Source: CAD feature listing. Evaluate the final solid. Frame: model axes, mm. A direction names the side the tool comes from. Round coordinates to 2 decimals unless told otherwise and drop trailing zeros. Loops run counter-clockwise (first coordinate to the right, second up) from the corner with the lowest first, then second, coordinate; pieces in that order, holes last. Notation, with made-up numbers: M -27,-9.5 L -22,-9.5 A23 cw -22,-0.5 Z; hole C 31.25,64.25 d6. An arc over 180 degrees is marked long. Answer as a JSON object with one key per item and string values.
from build123d import *

# Parameters (mm, degrees)
SKETCH_1_R      = 3
EXTRUDE_1_DEPTH = 5
SKETCH_2_R      = 3
EXTRUDE_2_DEPTH = 5


with BuildPart() as part:
    # 草图1 → 凸台-拉伸1 (new body)
    with BuildSketch(Plane(origin=(0, 0, 0), x_dir=(1, 0, 0), z_dir=(0, 1, 0))):
        with BuildLine():
            Line((-92.110125605, 6.217636835), (157.889874395, 6.217636835))
            ThreePointArc((157.889874395, 6.217636835), (162.889874395, 1.217636835), (157.889874395, -3.782363165))
            Line((157.889874395, -3.782363165), (-92.110125605, -3.782363165))
            ThreePointArc((-92.110125605, -3.782363165), (-97.110125605, 1.217636835), (-92.110125605, 6.217636835))
        make_face()
        with Locations(Location((-92.110125605, 1.217636835, 0), (0, 0, 270))):
            Circle(SKETCH_1_R, mode=Mode.SUBTRACT)
    extrude(amount=EXTRUDE_1_DEPTH)

    # 草图2 → 凸台-拉伸2 (add)
    with BuildSketch(Plane(origin=(0, 5, 0), x_dir=(1, 0, 0), z_dir=(0, 1, 0))):
        with Locations(Location((157.889874395, 1.217636835, 0), (0, 0, 270))):
            Circle(SKETCH_2_R)
    extrude(amount=EXTRUDE_2_DEPTH)


solid = part.part
Item 1: Contact query for a flat-ended pin moving along its axis: pin 1 Ø1 at (x, z) = (126, -0.5) entering from +Y. Output: stop coordinate, or through.
Answer sheet:
{"pin 1": "stops at y = 5"}
Item 2: Pull-direction query (Z, two-part tool) for faces 3 (the flat face through (158, 10, -1)), 4 (the flat face through (31, 2, -6.218)), 5 (the cylindrical face through (-93.936, 2.465, -3.598)); classes: pulls with the +Z half, pulls with the -Z half, needs draft (parallel to the pull), parting line crosses it, or undercut.
Answer sheet:
{"face 3": "needs draft", "face 4": "pulls with the -Z half", "face 5": "undercut"}
Item 3: Access query for faces 1 (the cylindrical face through (160.419, 7.465, 0.395)), 2 (the flat face through (35, 2, 3.782)). Directions: +Z, -Z, +X, -X, +Y, -Y. A direction counts if a zero-diameter tool reaches every point of the face in a straight line with its end or side. Return the directions, or none.
Answer sheet:
{"face 1": "+Y", "face 2": "+Z, +X, -X, +Y, -Y"}
Item 4: Section A-A on y = 3.25. Return the cut outline in (x, z).
Answer sheet:
{"outline": "M -92.11,-6.22 L 157.89,-6.22 A5 ccw 157.89,3.78 L -92.11,3.78 A5 ccw Z; hole C -92.11,-1.22 d6"}
Item 5: Line query: probe 1 along Y at (x, z) = (-48.5, 2.75); probe 2 along X at (y, z) = (1, -3.75); probe 3 along X at (y, z) = (2.25, -2.75). Output: solid intervals per line, ascending. Write a range as from..to.
Answer sheet:
{"probe 1": "y = 0..5", "probe 2": "x = -96.42..-93.72, -90.5..162.2", "probe 3": "x = -96.87..-94.69, -89.53..162.65"}
Item 6: Section B-B on x = 86. Return the cut outline in (y, z).
Answer sheet:
{"outline": "M 0,-6.22 L 5,-6.22 L 5,3.78 L 0,3.78 Z"}
